Job drawing, mm, ordinate dimensions from the low corner. One solid piece. Give positions to 0.01 mm unless a question says otherwise; leave off trailing zeros. Loops run counter-clockwise (first coordinate to the right, second up) from the corner with the lowest first, then second, coordinate; pieces in that order, holes last. Notation, with made-up numbers: M 71,14.25 L 104,14.25 A13 cw 104,21.25 Z; hole C -35.5,56.5 d2. An arc over 180 degrees is marked long. One line per question, with ' | ' between items.
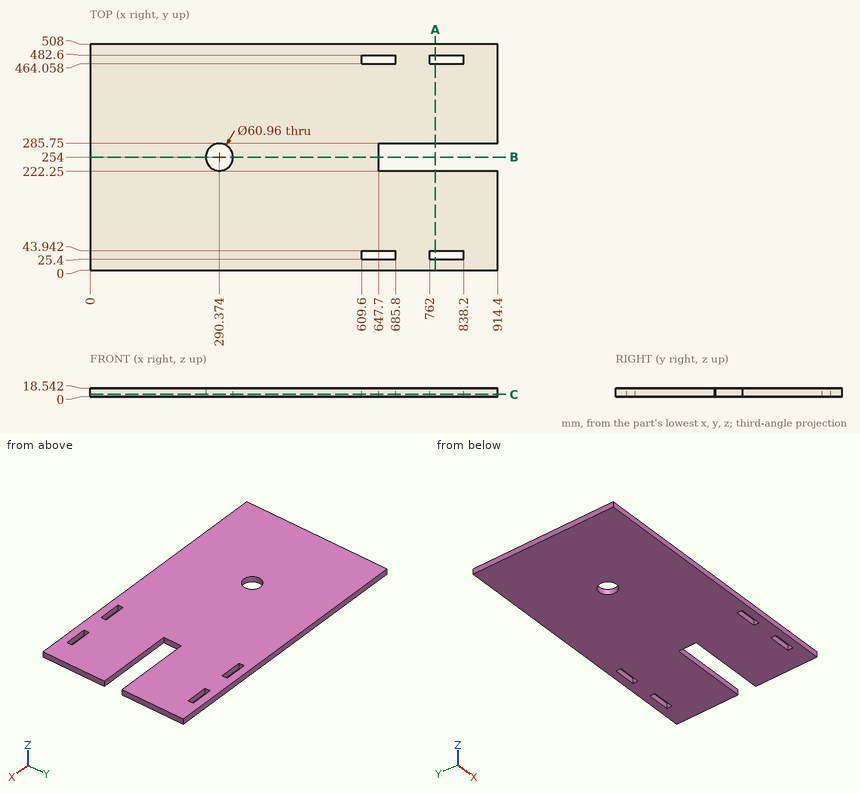
Item 1: Saw through at B-B on y = 254. Give the cut face in (x, z), and give its area (3 significant figures).
Conclusion:
outline: M 0,0 L 259.89,0 L 259.89,18.54 L 0,18.54 Z; M 320.85,0 L 647.7,0 L 647.7,18.54 L 320.85,18.54 Z | area: 10,900 mm²
Item 2: Saw through at A-A on x = 775. Give the cut face in (y, z).
Conclusion:
outline: M 0,0 L 25.4,0 L 25.4,18.54 L 0,18.54 Z; M 43.94,0 L 222.25,0 L 222.25,18.54 L 43.94,18.54 Z; M 285.75,0 L 464.06,0 L 464.06,18.54 L 285.75,18.54 Z; M 482.6,0 L 508,0 L 508,18.54 L 482.6,18.54 Z
Item 3: Drill centre lines: line 1 along Y through (x, z) = (664, 3.5); line 2 along X through (y, z) = (223, 3.75); line 3 along X through (y, z) = (228, 15.5) (1 decimal). Where is each one in solid material? Low to high. Write a range as [from, to].
Conclusion:
line 1: [0, 25.4], [43.94, 222.25], [285.75, 464.06], [482.6, 508] | line 2: [0, 647.7] | line 3: [0, 274.5], [306.3, 647.7]
Item 4: Saw through at C-C on z = 5. Give the cut face in (x, y).
Conclusion:
outline: M 0,0 L 914.4,0 L 914.4,222.25 L 647.7,222.25 L 647.7,285.75 L 914.4,285.75 L 914.4,508 L 0,508 Z; hole C 290.37,254 d60.96; hole M 609.6,25.4 L 685.8,25.4 L 685.8,43.94 L 609.6,43.94 Z; hole M 609.6,464.06 L 685.8,464.06 L 685.8,482.6 L 609.6,482.6 Z; hole M 762,25.4 L 838.2,25.4 L 838.2,43.94 L 762,43.94 Z; hole M 762,464.06 L 838.2,464.06 L 838.2,482.6 L 762,482.6 Z
